Build history of the part. All positions in model axes, mm. Face numbers are marked on the shaded views. Round coordinates to 2 decimals unless told otherwise and drop trailing zeros. Loops run counter-clockwise (first coordinate to the right, second up) from the corner with the lowest first, then second, coordinate; pieces in that order, holes last. Notation, with made-up numbers: M 32.5,29 L 86.5,29 A36 ccw 86.5,65 Z; hole C -2.5,7.25 d7. An arc over 180 degrees is marked long. Use one line per item in the form item = value. Start each with the question number.
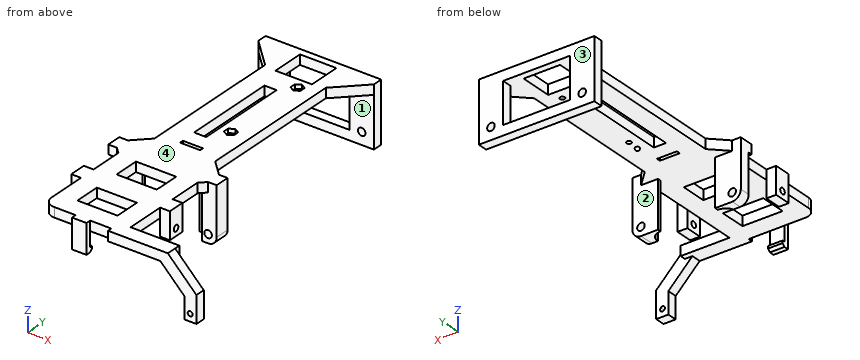
```python
from build123d import *

# Parameters (mm, degrees)
EXTRUDE_1_DEPTH     = 4
SKETCH_2_W          = 15
SKETCH_2_H          = 13.3866
CUT_EXTRUDE_1_DEPTH = 121.91505324
SKETCH_3_W          = 10
SKETCH_3_H          = 10
SKETCH_3_R          = 1.55
SKETCH_3_H_2        = 14.755
EXTRUDE_2_DEPTH     = 4
EXTRUDE_3_DEPTH     = 4
EXTRUDE_4_DEPTH     = 4
SKETCH_7_W          = 27.52
SKETCH_7_H          = 4
EXTRUDE_5_DEPTH     = 4
SKETCH_8_W          = 24.546067812
SKETCH_8_H          = 6.33
EXTRUDE_6_DEPTH     = 4
SKETCH_11_W         = 16.52
SKETCH_11_H         = 10.61
CUT_EXTRUDE_2_DEPTH = 132.394668556
SKETCH_12_W         = 11
SKETCH_12_H         = 6.89
SKETCH_12_R         = 1.25
EXTRUDE_6711_DEPTH  = 4
SKETCH_14_R         = 1
CUT_EXTRUDE_3_DEPTH = 131.700110654
SKETCH_15_R         = 0.9
EXTRUDE_9_DEPTH     = 1
FILLET_1_R          = 0.9
CUT_EXTRUDE_START   = -1.7
SKETCH_16_R         = 1
CUT_EXTRUDE_4_DEPTH = 1.7
CUT_EXTRUDE_5_DEPTH = 131.700110654
SKETCH_19_W         = 5
SKETCH_19_H         = 38.5268
SKETCH_19_W_2       = 8.236887868
SKETCH_19_H_2       = 1.55
CUT_EXTRUDE_6_DEPTH = 131.700110654
EXTRUDE_12_DEPTH    = 23.28
CUT_EXTRUDE_7_REACH = 99.296
SKETCH_23_R         = 1.55
EXTRUDE_13_DEPTH    = 4
CUT_EXTRUDE_START_2 = -19.28
CUT_EXTRUDE_8_DEPTH = 19.48
SKETCH_26_W         = 10.1
SKETCH_26_H         = 2
EXTRUDE_14_DEPTH    = 3


# Read off the part's stored shape, not the designer's step: the extrude step
with BuildPart() as part:
    # Sketch 1 → Extrude 1 (new body)
    with BuildSketch(Plane.XY):
        with BuildLine():
            Line((-16.26, -7.25), (-16.26, 119.75))
            Line((-16.26, 119.75), (16.26, 119.75))
            Line((16.26, 119.75), (16.26, -7.25))
            ThreePointArc((16.26, -7.25), (14.939051583, -10.439051583), (11.75, -11.76))
            Line((11.75, -11.76), (-11.75, -11.76))
            ThreePointArc((-11.75, -11.76), (-14.939051583, -10.439051583), (-16.26, -7.25))
        make_face()
    extrude(amount=EXTRUDE_1_DEPTH)

    # Sketch 2 → Cut-Extrude 1 (cut, through all)
    with BuildSketch(Plane(origin=(0, 0, 0), x_dir=(-1, 0, 0), z_dir=(0, 0, -1))):
        with Locations((0, 110.2067)):
            Rectangle(SKETCH_2_W, SKETCH_2_H)
    extrude(amount=-CUT_EXTRUDE_1_DEPTH, mode=Mode.SUBTRACT)

    # Sketch 3 → Extrude 2 (add)
    # profile 1 of 2: a face of its own
    with BuildSketch(Plane(origin=(0, 119.75, 0), x_dir=(1, 0, 0), z_dir=(0, 1, 0))):
        with Locations((-18.76, 15.755)):
            Rectangle(SKETCH_3_W, SKETCH_3_H)
        with Locations(Location((-18.76, 15.755, 0), (0, 0, 270))):
            Circle(SKETCH_3_R, mode=Mode.SUBTRACT)
    # profile 2 of 2: a face of its own
    with BuildSketch(Plane(origin=(0, 119.75, 0), x_dir=(1, 0, 0), z_dir=(0, 1, 0))):
        with Locations((-18.76, 3.3775)):
            Rectangle(SKETCH_3_W, SKETCH_3_H_2)
    extrude_2 = extrude(amount=-EXTRUDE_2_DEPTH)

    # Mirror 1: Extrude 2 across plane
    add(extrude_2.mirror(Plane(origin=(0, 0, 0), x_dir=(0, 0, 1), z_dir=(1, 0, 0))))

    # Sketch 6 → Extrude 4 (add)
    with BuildSketch(Plane.XY.offset(4)):
        Polygon((-16.26, 115.75), (-23.76, 115.75), (-16.26, 108.25), align=None)
        Polygon((16.26, 115.75), (16.26, 108.25), (23.76, 115.75), align=None)
    extrude(amount=-EXTRUDE_4_DEPTH)

    # Sketch 7 → Extrude 5 (add)
    with BuildSketch(Plane(origin=(0, 119.75, 0), x_dir=(1, 0, 0), z_dir=(0, 1, 0))):
        with Locations((0, 18.755)):
            Rectangle(SKETCH_7_W, SKETCH_7_H)
    extrude(amount=-EXTRUDE_5_DEPTH)



with BuildPart() as body_2:
    # Sketch 5 → Extrude 3 (new body)
    with BuildSketch(Plane(origin=(0, -13.58, 0), x_dir=(1, 0, 0), z_dir=(0, 1, 0))):
        Polygon((47.78, 9.855), (43.08, 9.855), (29.225, -4), (36.296067812, -4), (48.08, 7.783932188), (48.08, 9.855), align=None)
        with BuildLine():
            Line((47.78, 18.755), (43.08, 18.755))
            Line((43.08, 18.755), (43.08, 9.855))
            Line((43.08, 9.855), (47.78, 9.855))
            Line((47.78, 9.855), (47.78, 15.105))
            Line((47.78, 15.105), (46.239934208, 15.105))
            ThreePointArc((46.239934208, 15.105), (44.48, 15.755), (46.239934208, 16.405))
            Line((46.239934208, 16.405), (47.78, 16.405))
            Line((47.78, 16.405), (47.78, 18.755))
        make_face()
        with BuildLine():
            Line((48.08, 18.755), (47.78, 18.755))
            Line((47.78, 18.755), (47.78, 16.405))
            Line((47.78, 16.405), (46.239934208, 16.405))
            ThreePointArc((46.239934208, 16.405), (46.418065618, 16.10145764), (46.48, 15.755))
            ThreePointArc((46.48, 15.755), (46.418065618, 15.40854236), (46.239934208, 15.105))
            Line((46.239934208, 15.105), (47.78, 15.105))
            Line((47.78, 15.105), (47.78, 9.855))
            Line((47.78, 9.855), (48.08, 9.855))
            Line((48.08, 9.855), (48.08, 18.755))
        make_face()
    extrude(amount=EXTRUDE_3_DEPTH)


with BuildPart() as part_1:
    add(part.part)

    add(body_2.part)  # Extrude 6 merges body 2
    # Sketch 8 → Extrude 6 (add)
    with BuildSketch(Plane.XY.offset(4)):
        with Locations((24.023033906, -10.415)):
            Rectangle(SKETCH_8_W, SKETCH_8_H)
    extrude(amount=-EXTRUDE_6_DEPTH)

    # Sketch 11 → Cut-Extrude 2 (cut, through all)
    with BuildSketch(Plane.XY.offset(4)):
        with Locations((0, 1.545)):
            Rectangle(SKETCH_11_W, SKETCH_11_H)
        with Locations((0, 22.955)):
            Rectangle(SKETCH_11_W, SKETCH_11_H)
    extrude(amount=-CUT_EXTRUDE_2_DEPTH, mode=Mode.SUBTRACT)

    # Sketch 12 → Extrude 6711 (add)
    with BuildSketch(Plane.ZY.offset(16.26)):
        with Locations((-1.5, 12.295)):
            Rectangle(SKETCH_12_W, SKETCH_12_H)
        with Locations((-4, 12.25)):
            Circle(SKETCH_12_R, mode=Mode.SUBTRACT)
    extrude_6711 = extrude(amount=EXTRUDE_6711_DEPTH)

    # Mirror 4: Extrude 6711 across plane
    add(extrude_6711.mirror(Plane(origin=(0, 0, 0), x_dir=(0, 0, 1), z_dir=(1, 0, 0))))

    # Sketch 14 → Cut-Extrude 3 (cut, through all)
    with BuildSketch(Plane(origin=(0, 0, 0), x_dir=(-1, 0, 0), z_dir=(0, 0, -1))):
        with Locations((-5, 62.6)):
            Circle(SKETCH_14_R)
        with Locations((-5, 99)):
            Circle(SKETCH_14_R)
    extrude(amount=-CUT_EXTRUDE_3_DEPTH, mode=Mode.SUBTRACT)

    # Sketch 15 → Extrude 9 (add)
    with BuildSketch(Plane(origin=(0, 0, 0), x_dir=(-1, 0, 0), z_dir=(0, 0, -1))):
        with Locations(Location((-5, 94.35, 0), (0, 0, 180))):
            Circle(SKETCH_15_R)
        with Locations(Location((-5, 57.98, 0), (0, 0, 180))):
            Circle(SKETCH_15_R)
    extrude(amount=EXTRUDE_9_DEPTH)

    # Fillet 1
    fillet_1_edges = [part_1.edges().sort_by_distance(p)[0] for p in [
        (4.1, 94.35, -1),
        (4.1, 57.98, -1),
    ]]
    fillet(fillet_1_edges, radius=FILLET_1_R)

    # Sketch 16 → Cut-Extrude 4 (cut)
    # profile 1 of 2: a face of its own
    with BuildSketch(Plane.XY.offset(4).offset(CUT_EXTRUDE_START)):
        Polygon((7.05, 61.416431948), (7.05, 63.783568052), (5, 64.967136104), (2.95, 63.783568052), (2.95, 61.416431948), (5, 60.232863896), align=None)
        with Locations(Location((5, 62.6, 0), (0, 0, 180))):
            Circle(SKETCH_16_R, mode=Mode.SUBTRACT)
    # profile 2 of 2: a face of its own
    with BuildSketch(Plane.XY.offset(4).offset(CUT_EXTRUDE_START)):
        Polygon((2.95, 97.816431948), (5, 96.632863896), (7.05, 97.816431948), (7.05, 100.183568052), (5, 101.367136104), (2.95, 100.183568052), align=None)
        with Locations(Location((5, 99, 0), (0, 0, 180))):
            Circle(SKETCH_16_R, mode=Mode.SUBTRACT)
    extrude(amount=CUT_EXTRUDE_4_DEPTH, mode=Mode.SUBTRACT)

    # Sketch 17 → Cut-Extrude 5 (cut, symmetric)
    with BuildSketch(Plane(origin=(0, 0, 0), x_dir=(-1, 0, 0), z_dir=(0, 0, -1))):
        Polygon((-12.5, 104.49), (-16.26, 108.25), (-16.26, 40.2266), (-12.5, 43.9866), align=None)
    cut_extrude_5 = extrude(amount=CUT_EXTRUDE_5_DEPTH, both=True, mode=Mode.SUBTRACT)

    # Mirror 2: Cut-Extrude 5 across plane
    add(cut_extrude_5.mirror(Plane(origin=(0, 0, 0), x_dir=(0, 0, 1), z_dir=(1, 0, 0))), mode=Mode.SUBTRACT)

    # Sketch 19 → Cut-Extrude 6 (cut, through all)
    with BuildSketch(Plane(origin=(0, 0, 0), x_dir=(-1, 0, 0), z_dir=(0, 0, -1))):
        with Locations((2, 74.25)):
            Rectangle(SKETCH_19_W, SKETCH_19_H)
        with Locations((0, 47.675)):
            Rectangle(SKETCH_19_W_2, SKETCH_19_H_2)
    extrude(amount=-CUT_EXTRUDE_6_DEPTH, mode=Mode.SUBTRACT)

    # Sketch 22 → Extrude 12 (add)
    with BuildSketch(Plane.XY.offset(4)):
        with BuildLine():
            Line((16.26, 32.704986911), (16.26, 31.75))
            Line((16.26, 31.75), (22.285, 31.75))
            Line((22.285, 31.75), (22.285, 37.75))
            Line((22.285, 37.75), (11.75, 37.75))
            Line((11.75, 37.75), (11.75, 36.36))
            ThreePointArc((11.75, 36.36), (14.652551493, 35.331521301), (16.26, 32.704986911))
        make_face()
    extrude_12 = extrude(amount=-EXTRUDE_12_DEPTH)

    # Sketch 23 → Cut-Extrude 7 (cut, up to next)
    with BuildSketch(Plane(origin=(0, 37.75, 0), x_dir=(1, 0, 0), z_dir=(0, 1, 0)), mode=Mode.PRIVATE) as cut_extrude_7_sk1:
        with Locations(Location((18.76, 15.755, 0), (0, 0, 270))):
            Circle(SKETCH_23_R)
    cut_extrude_7_tool1 = extrude(cut_extrude_7_sk1.sketch, amount=-CUT_EXTRUDE_7_REACH, mode=Mode.PRIVATE) & part_1.part
    # Sketch 23 → Cut-Extrude 7 (cut, up to next)
    with BuildSketch(Plane(origin=(0, 37.75, 0), x_dir=(1, 0, 0), z_dir=(0, 1, 0)), mode=Mode.PRIVATE) as cut_extrude_7_sk2:
        with BuildLine():
            ThreePointArc((18.76, 19.28), (21.252551404, 18.247551404), (22.285, 15.755))
            Line((22.285, 15.755), (22.285, 19.28))
            Line((22.285, 19.28), (18.76, 19.28))
        make_face()
    cut_extrude_7_tool2 = extrude(cut_extrude_7_sk2.sketch, amount=-CUT_EXTRUDE_7_REACH, mode=Mode.PRIVATE) & part_1.part
    cut_extrude_7_1 = cut_extrude_7_tool1.solids().sort_by_distance((18.76, 37.75, -15.755))[0]
    add(cut_extrude_7_1, mode=Mode.SUBTRACT)
    cut_extrude_7_2 = cut_extrude_7_tool2.solids().sort_by_distance((21.497628, 37.75, -18.492628))[0]
    add(cut_extrude_7_2, mode=Mode.SUBTRACT)
    cut_extrude_7 = cut_extrude_7_1 + cut_extrude_7_2  # Cut-Extrude 7 as one shape, for the pattern or mirror that repeats it

    # Sketch 24 → Extrude 13 (add)
    with BuildSketch(Plane.XY.offset(4)):
        Polygon((16.26, 40.2266), (18.7366, 37.75), (18.7366, 31.75), (16.26, 29.2734), align=None)
    extrude_13 = extrude(amount=-EXTRUDE_13_DEPTH)

    # Mirror 3: Extrude 12, Cut-Extrude 7, Extrude 13 across plane
    add(extrude_12.mirror(Plane(origin=(0, 0, 0), x_dir=(0, 0, 1), z_dir=(1, 0, 0))))
    add(cut_extrude_7.mirror(Plane(origin=(0, 0, 0), x_dir=(0, 0, 1), z_dir=(1, 0, 0))), mode=Mode.SUBTRACT)
    add(extrude_13.mirror(Plane(origin=(0, 0, 0), x_dir=(0, 0, 1), z_dir=(1, 0, 0))))

    # Cut-Extrude 8 outline → Cut-Extrude 8 (cut)
    with BuildSketch(Plane.XY.offset(CUT_EXTRUDE_START_2)):
        with BuildLine():
            ThreePointArc((-16.26, 31.75), (-16.176051621, 32.616121846), (-15.927331684, 33.45))
            Line((-15.927331684, 33.45), (-22.285, 33.45))
            Line((-22.285, 33.45), (-22.285, 31.75))
            Line((-22.285, 31.75), (-16.26, 31.75))
        make_face()
    extrude(amount=CUT_EXTRUDE_8_DEPTH, mode=Mode.SUBTRACT)

    # Sketch 26 → Extrude 14 (add, symmetric)
    with BuildSketch(Plane(origin=(0, 0, 0), x_dir=(0, 0, -1), z_dir=(1, 0, 0))):
        with Locations((1.05, -12.76)):
            Rectangle(SKETCH_26_W, SKETCH_26_H)
        Polygon((8.1, -11.76), (8.1, -13.76), (6.1, -13.76), (6.1, -11.76), (6.1, -10.76), (7.1, -10.76), align=None)
    extrude(amount=EXTRUDE_14_DEPTH, both=True)


solid = part_1.part
```
Q1. Pull direction Y, two halves, no side cores. Call the marked faces 1, 2, 3 and 4: pulls with the +Y half, pulls with the -Y half, needs draft (parallel to the pull), parting line crosses it, or undercut.
Q2. Drop flat-ended pins along their axis: P1, Ø10, axis at y = 14, z = -11.5, coming from the +X side; P2, Ø6.5, axis at x = 14, y = 36, coming from the -Z side; P3, Ø3, axis at x = -18.5, z = 0, coming from the -Y side; P4, Ø5, axis at x = -0.5, z = -9, coming from the -Y side. Give the stop position or say it passes through.
Q3. Saw through at B-B (x = -1.5). Give the number of separate pieces and of enclosed holes in the cut face, and give its area (3 significant figures).
Q4. Saw through at A-A (y = -1). Give the cut face in (x, z).
Q5. Saw through at C-C (x = 10). Give the cut face in (y, z) (3 decimals).
Q6. Wall check: probe 1 along Y at (x, z) = (-17.8, -4); probe 2 along Y at (x, z) = (17.15, -4); probe 3 along X at (y, z) = (14, -6). Give the ranges that are in metal, low to high.
Q7. Saw through at D-D (y = 39.5). Give the cut face in (x, z).
Filled in:
q1.face_1 = undercut
q1.face_2 = undercut
q1.face_3 = pulls with the +Y half
q1.face_4 = needs draft
q2.P1 = 20.26
q2.P2 = -19.28
q2.P3 = 8.85
q2.P4 = -13.76
q3.separate_pieces = 7
q3.enclosed_holes = 0
q3.area = 269 mm²
q4.outline = M -16.26,0 L -8.26,0 L -8.26,4 L -16.26,4 Z; M 8.26,0 L 16.26,0 L 16.26,4 L 8.26,4 Z
q5.outline = M -11.76,0 L 119.75,0 L 119.75,4 L -11.76,4 Z; M 115.75,-20.755 L 119.75,-20.755 L 119.75,-16.755 L 115.75,-16.755 Z
q6.probe_1 = 8.85 to 11, 13.5 to 15.74, 33.45 to 37.75, 115.75 to 119.75
q6.probe_2 = 8.85 to 11, 13.5 to 15.74, 31.75 to 37.75, 115.75 to 119.75
q6.probe_3 = -20.26 to -16.26, 16.26 to 20.26
q7.outline = M -16.99,0 L 16.99,0 L 16.99,4 L -16.99,4 Z
